Autodesk Fusion 360 part; units mm, degrees
sketch "Sketch1" plane through (0, 0, 0) normal (0, 0, 1) x (1, 0, 0)
  line L0 (0, 0) -> (34.55, 0)
  line L1 (34.55, 0) -> (34.55, 6.8)
  line L2 (15.6, 0) -> (15.6, 9.67) construction
  line L3 (34.55, 6.8) -> (15.6, 9.67)
  line L4 (5.05, 0) -> (5.05, 8.6) construction
  line L5 (15.6, 9.67) -> (5.05, 8.6)
  line L6 (0, 0) -> (0, 14.12)
  line L7 (0, 14.12) -> (3.475, 14.12)
  spline S0 degree 2 poles (3.475, 14.12) (4.5, 9.5) (5.05, 8.6) knots 0 0 0 0.575587 0.575587 0.575587 weights 1 2.082456 1
  line L8 (3.125, 0) -> (3.125, 5.7)
  line L9 (3.125, 5.7) -> (0, 5.7)
  line L10 (13.66, 0) -> (13.66, 1.45) construction
  spline S1 degree 2 poles (3.125, 5.7) (6, 1.5) (13.66, 1.45) knots 0 0 0 1.170983 1.170983 1.170983
  line L11 (13.66, 1.45) -> (14.4767, 0)
  line L12 (1.16, 0) -> (1.16, 14.12)
  dimension "d1" = 34.55
  dimension "d2" = 6.8
  dimension "d3" = 9.67
  dimension "d4" = 15.6
  dimension "d5" = 8.6
  dimension "d6" = 5.05
  dimension "d7" = 14.12
  dimension "d8" = 3.475
  dimension "d9" = 3.125
  dimension "d10" = 5.7
  dimension "d11" = 1.45
  dimension "d12" = 13.66
  dimension "d13" = 1.16
revolve "Revolve1" add sketch "Sketch1" angle 360 about axis through (0, 0, 0) along (0, 1, 0) contours L0 L8 L9 L12 | L0 L1 L3 L5 L7 S0 L9 S1 L11 L12
sketch "Sketch2" plane through (0, 0, 0) normal (0, -1, 0) x (1, 0, 0)
  circle A0 centre (0, 0) radius 3.125
  circle A1 centre (0, 0) radius 1.16
  line L0 (1, 2.9607) -> (1, 14.4421)
  circle A2 centre (0, 0) radius 34.55
  circle A3 centre (0, 0) radius 14.4767
  line L1 (-1, 14.4421) -> (-1, 2.9607)
  line L2 (0, 3.125) -> (0, 14.4767) construction
  line L3 (0, 0) -> (0, 3.125) construction
  dimension "d15" = 2
extrude "Extrude1" add sketch "Sketch2" against normal blind 7 contours A0 L0 A3 L1 picked at (-10.6389, -0.7571)
pattern_circular "C-Pattern1" count 4 over 360 about axis through (0, 5.7, 0) along (0, -1, 0) of "Extrude1"
equation "d1 = ( 69.1 / 2 ) * 1 mm"
equation "d4 = ( 31.2 / 2 ) * 1 mm"
equation "d6 = ( 10.1 / 2 ) * 1 mm"
equation "d8 = ( 6.95 / 2 ) * 1 mm"
equation "d9 = ( 6.25 / 2 ) * 1 mm"
equation "d12 = ( 27.32 / 2 ) * 1 mm"
equation "d13 = ( 2.32 / 2 ) * 1 mm"
Input: part model. Units: mm. Frame: model coordinates. Round coordinates to 2 decimals unless told otherwise and drop trailing zeros. Loops run counter-clockwise (first coordinate to the right, second up) from the corner with the lowest first, then second, coordinate; pieces in that order, holes last. Notation, with made-up numbers: (-5, 79.25) -> (16, 79.25) arc R12 cw to (16, 86.25) -> close; hole circle Ø7 at (-7.5, 1.5). An arc over 180 degrees is marked (long way). One line per item, written item: value.
(1) Mould query, pull axis Z, two halves, no side actions, for faces 1 (the face through (1.072, 7.159, 0.444)), 2 (the face through (16.01, 9.49, 5.04)), 3 (the face through (0, 0, 7)). Classes: pulls with the +Z half, pulls with the -Z half, needs draft (parallel to the pull), parting line crosses it, or undercut.
Geometry check:
face 1: undercut
face 2: parting line crosses it
face 3: needs draft
(2) Pin query (flat end, axial travel): pin 1 (6 mm diameter, centred on x = 24.5, z = 5.5, fed in from +Y); pin 2 (1 mm diameter, centred on x = 10, z = 4.5, fed in from +Y); pin 3 (8 mm diameter, centred on x = 19.5, y = 4, fed in from -Z); pin 4 (8 mm diameter, centred on x = -26.5, z = 20.5, fed in from -Y). Return the tip coordinate at first contact, or that it passes through.
Geometry check:
pin 1: y = 8.68
pin 2: y = 9.25
pin 3: z = -30.88
pin 4: y = 0
(3) Section A-A (y = 4.25). Return the cut outline in (x, z).
Geometry check:
outline: circle Ø69.1 at (0, 0); hole circle Ø2.32 at (0, 0)
(4) Material intervals for line 1 (X direction, y = 3.5, z = 0); line 2 (Z direction, x = 0, y = 10.5); line 3 (X direction, y = 11.5, z = 0), sorted ascending. Write a range as [from, to].
Geometry check:
line 1: [-34.55, -1.16], [1.16, 34.55]
line 2: [-4.32, -1.16], [1.16, 4.32]
line 3: [-4.07, -1.16], [1.16, 4.07]
